Read the model definition and answer for the solid it produces. Units are mm, in the model's axes. Face numbers are marked on the shaded views. A direction names the side the tool comes from. Coordinates: 2 decimals unless noted, no trailing zeros. Write each loop counter-clockwise with the first axis right and the second up, starting at its lowest first coordinate (ties: lowest second). Pieces come first, ordered by that corner, then holes. Notation, with made-up numbers: (0, 22) -> (25, 22) arc R22 cw to (25, 40) -> close; hole circle Ø3 at (53.25, -29.5). An arc over 180 degrees is marked (long way). Answer as a JSON object with one key per item and string values. Group by question number.
(1) Find section C-C (z = 21). Give the vertices of the cut face in (x, y).
(2) Find section B-B (x = -18). Give the vertices of the cut face in (y, z), then the cut area to 3 significant figures.
(3) Flat-ended cylindrical pins translate along their axes: P1, Ø10, axis at y = -5, z = 33, coming from the +X side; P2, Ø5, axis at x = -8, z = 62, coming from the -Y side. Find the tip coordinate at first contact, or state that the pin passes through.
(4) Which of the six approach directions +Z, -Z, +X, -X, +Y, -Y give full straight-line access (tool end or side, diameter ignored) to the marked faces 4, 5 and 6?
(5) Straight lines are drawn through the part: L1, parallel to Z at x = -36, y = 15.5; L2, parallel to X at y = 0, z = 52; L3, parallel to Y at x = 25.5, z = 17.5. For each, find the intervals that lie inside material, in ascending order.
(6) For a pull along X with two mould halves and no side action, classify the marked faces 1, 2 and 3 as +X half, -X half, draft (parallel to the pull), parting line (faces both ways), or undercut.
(7) Find section A-A (y = -22.5). Give the vertices of the cut face in (x, z).
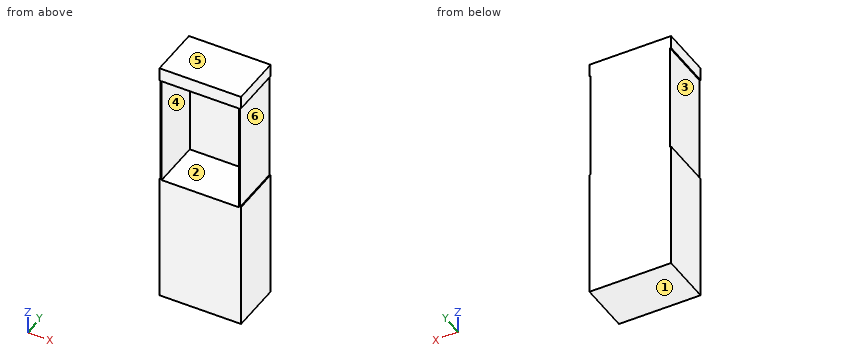
from build123d import *

# Parameters (mm, degrees)
F0_W     = 87.7677612007
F0_H     = 270.8992287517
F0_W_2   = 82.2834707797
F0_H_2   = 132.241293788
F1_DEPTH = 27.94
F2_W     = 83.075709641
F2_H     = 117.8717985749
F3_DEPTH = 53.34
F4_W     = 55.88
F4_H     = 117.8577281535
F5_DEPTH = 1.016
F6_W     = 55.88
F6_H     = 117.6069006324
F7_DEPTH = 1.016


with BuildPart() as f1:
    # F0 (on Front) → F1 (new body, symmetric)
    with BuildSketch(Plane.XZ):
        with Locations((-2.0966473967, -40.4195971787)):
            Rectangle(F0_W, F0_H)
        with Locations((-2.0786840469, 17.0819833875)):
            Rectangle(F0_W_2, F0_H_2, mode=Mode.SUBTRACT)
        with Locations((-2.0786840469, 17.0819833875)):
            Rectangle(F0_W_2, F0_H_2)
    extrude(amount=F1_DEPTH, both=True)

    # F2 (on face) → F3 (cut)
    with BuildSketch(Plane.XZ.offset(27.94)):
        with Locations((-2.0913966, 21.4343853295)):
            Rectangle(F2_W, F2_H)
    extrude(amount=-F3_DEPTH, mode=Mode.SUBTRACT)

    # F4 (on face) → F5 (cut)
    with BuildSketch(Plane.YZ.offset(41.7872332036)):
        with Locations((0, 22.4192347378)):
            Rectangle(F4_W, F4_H)
    extrude(amount=-F5_DEPTH, mode=Mode.SUBTRACT)

    # F6 (on face) → F7 (cut)
    with BuildSketch(Plane(origin=(-45.980527997, 0, 0), x_dir=(0, -1, 0), z_dir=(-1, 0, 0))):
        with Locations((0, 22.0092870295)):
            Rectangle(F6_W, F6_H)
    extrude(amount=-F7_DEPTH, mode=Mode.SUBTRACT)


solid = f1.part
Results below:
{
 "1": {"outline": "(-44.96, -27.94) -> (-43.63, -27.94) -> (-43.63, 25.4) -> (39.45, 25.4) -> (39.45, -27.94) -> (40.77, -27.94) -> (40.77, 27.94) -> (-44.96, 27.94) -> close"},
 "2": {"outline": "(-27.94, -175.87) -> (27.94, -175.87) -> (27.94, 95.03) -> (-27.94, 95.03) -> (-27.94, 80.37) -> (25.4, 80.37) -> (25.4, -37.5) -> (-27.94, -37.5) -> close", "area": "8,850 mm2"},
 "3": {"P1": "stops at x = 40.77", "P2": "stops at y = 25.4"},
 "4": {"face 4": "-Y", "face 5": "+Z, +X, -X, +Y, -Y", "face 6": "+X, +Y, -Y"},
 "5": {"L1": "z = -175.87 to -37.5, 80.37 to 95.03", "L2": "x = -44.96 to -43.63, 39.45 to 40.77", "L3": "y = 25.4 to 27.94"},
 "6": {"face 1": "draft", "face 2": "undercut", "face 3": "-X half"},
 "7": {"outline": "(-45.98, -175.87) -> (41.79, -175.87) -> (41.79, -36.51) -> (40.77, -36.51) -> (40.77, 81.35) -> (41.79, 81.35) -> (41.79, 95.03) -> (-45.98, 95.03) -> (-45.98, 80.81) -> (-44.96, 80.81) -> (-44.96, -36.79) -> (-45.98, -36.79) -> close; hole (-43.63, -37.5) -> (39.45, -37.5) -> (39.45, 80.37) -> (-43.63, 80.37) -> close"}
}
